Part model, mm, in its own coordinate system. Coordinates: 2 decimals unless noted, no trailing zeros. Loops run counter-clockwise (first coordinate to the right, second up) from the corner with the lowest first, then second, coordinate; pieces in that order, holes last. Notation, with made-up numbers: M -34.75,-38.5 L 0.25,-38.5 A28 ccw 0.25,-6.5 Z; hole C -34,14 d3. An arc over 180 degrees is marked long. Answer as a JSON object with one key per item and string values. Group by question number.
1. Drop flat-ended pins along their axis: pin 1 Ø1.9 at (y, z) = (1, 39) entering from +X (3 decimals); pin 2 Ø1.9 at (x, z) = (-1, 44) entering from -Y (3 decimals); pin 3 Ø0.5 at (y, z) = (8.5, 77.5) entering from -X. Give the stop position or say it passes through.
2. Saw through at A-A on y = 0. Write the cut outline in (x, z) (3 decimals), then the cut area to 3 significant figures.
3. Drill centre lines: L1, parallel to Y at x = 0, z = 90 (3 decimals); L2, parallel to Y at x = 7.25, z = 91.5; L3, parallel to Y at x = -5, z = 58. Where is each one in solid material? Low to high.
from build123d import *

# Parameters (mm, degrees)
SKETCH1_R           = 2.5
BOSS_EXTRUDE1_DEPTH = 114
FILLET1_R           = 2


with BuildPart() as part:
    # Sketch1 → Boss-Extrude1 (new body)
    with BuildSketch(Plane.XY):
        Polygon((-5.46, -6.42), (-3.215, -4.175), (3.215, -4.175), (5.46, -6.42), (5.46, -8.22), (3.06, -8.22), (3.06, -10), (10, -10), (10, -3.06), (8.22, -3.06), (8.22, -5.46), (6.42, -5.46), (4.175, -3.215), (4.175, 3.215), (6.42, 5.46), (8.22, 5.46), (8.22, 3.06), (10, 3.06), (10, 10), (3.06, 10), (3.06, 8.22), (5.46, 8.22), (5.46, 6.42), (3.215, 4.175), (-3.215, 4.175), (-5.46, 6.42), (-5.46, 8.22), (-3.06, 8.22), (-3.06, 10), (-10, 10), (-10, 3.06), (-8.22, 3.06), (-8.22, 5.46), (-6.42, 5.46), (-4.175, 3.215), (-4.175, -3.215), (-6.42, -5.46), (-8.22, -5.46), (-8.22, -3.06), (-10, -3.06), (-10, -10), (-3.06, -10), (-3.06, -8.22), (-5.46, -8.22), align=None)
        with Locations(Location((0, 0, 0), (0, 0, 180))):
            Circle(SKETCH1_R, mode=Mode.SUBTRACT)
    extrude(amount=BOSS_EXTRUDE1_DEPTH)

    # Fillet1
    fillet1_edges = [part.edges().sort_by_distance(p)[0] for p in [
        (10, -10, 57),
        (-10, -10, 57),
        (-10, 10, 57),
        (10, 10, 57),
    ]]
    fillet(fillet1_edges, radius=FILLET1_R)


solid = part.part
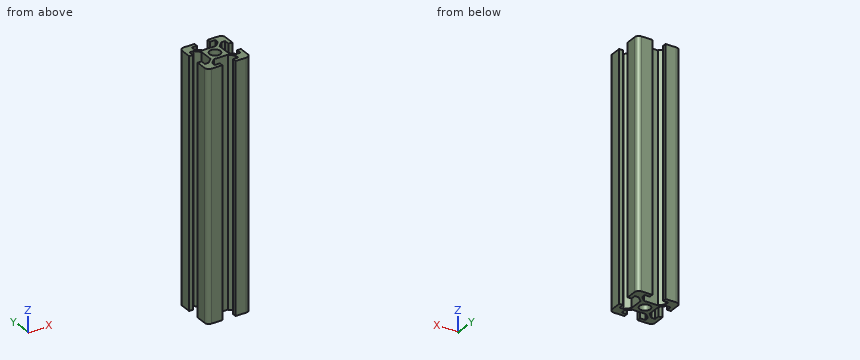
Outcome:
{
 "1": {"pin 1": "stops at x = 4.175", "pin 2": "stops at y = -4.175", "pin 3": "stops at x = -9.98"},
 "2": {"outline": "M -4.175,0 L -2.5,0 L -2.5,114 L -4.175,114 Z; M 2.5,0 L 4.175,0 L 4.175,114 L 2.5,114 Z", "area": "382 mm²"},
 "3": {"L1": "y = -4.175 to -2.5, 2.5 to 4.175", "L2": "y = -10 to -5.46, 5.46 to 10", "L3": "y = -10 to -8.22, -5.96 to -4.04, 4.04 to 5.96, 8.22 to 10"}
}
